Verification items for the finished model (mm, model axes). Face numbers are marked on the shaded views. Coordinates: 2 decimals unless noted, no trailing zeros. Order: outer loops, then holes, each group sorted by start corner. A loop starts at its lowest first (then second) coordinate and runs counter-clockwise, first axis right, second up. Notation, with made-up numbers: M 36,46.25 L 87,46.25 A17 ccw 87,62.25 Z; hole C -16.75,-27.5 d9. An arc over 180 degrees is marked long. Return JSON: item names as keys, results as strings. Group by question number.
Q1. Thickness scan on probe 1 along Z at (x, y) = (3, 23.5); probe 2 along Z at (x, y) = (-28, 0); probe 3 along Z at (x, y) = (22, -13.5). Record the ranges inside material, lowest first.
Q2. Section check A-A, the plane y = 0. Count the separate pieces of the cut face and the enclosed holes in it, then the cut area to 3 significant figures.
Q3. Go/stop test with flat-tipped pins: pin 1 Ø1.4 at (y, z) = (7.5, 54) entering from -X (3 decimals); pin 2 Ø2.5 at (y, z) = (20.5, -222) entering from -X; pin 3 Ø3.5 at (x, y) = (-1.5, 8.5) entering from +Z. Record where each tip stops, or that it passes through.
Q4. Mould release check, pull along Z, two halves, no side actions. Record for the marked faces 1 and 2: pulls with the +Z half, pulls with the -Z half, needs draft (parallel to the pull), parting line crosses it, or undercut.
Q5. Section check B-B, the plane y = 25.4. Enter the section's corners in (x, z).
Q6. Section check D-D, the plane z = -266.5. Enter the section's corners in (x, y), then the cut area to 3 significant figures.
Q7. Section check C-C, the plane z = -370.5. Enter the section's corners in (x, y) (3 decimals).
from build123d import *

# Parameters (mm, degrees)
BOSS_EXTRUDE1_DEPTH   = 5.08
LPATTERN1_COUNT       = 2
LPATTERN1_PITCH       = 104.14
SKETCH2_R             = 6.35
BOSS_EXTRUDE2_DEPTH   = 104.14
LPATTERN2_COUNT       = 3
LPATTERN2_PITCH       = 114.3
BODY_MOVE_COPY1_ANGLE = 120
BODY_MOVE_COPY2_ANGLE = 120
SKETCH3_R             = 12.7
BOSS_EXTRUDE3_DEPTH   = 5.08
BOSS_EXTRUDE4_START   = 114.3
SKETCH3_2_R           = 12.7
BOSS_EXTRUDE4_DEPTH   = 5.08
SKETCH4_R             = 6.985
BOSS_EXTRUDE5_DEPTH   = 76.2
SKETCH5_R             = 6.35
BOSS_EXTRUDE6_DEPTH   = 76.2
BOSS_EXTRUDE7_START   = 5.499261
SKETCH6_W             = 6.35
SKETCH6_H             = 25.4
BOSS_EXTRUDE7_DEPTH   = 4.660739


with BuildPart() as part:
    # Sketch1 → Boss-Extrude1 (new body)
    with BuildSketch(Plane.XY):
        with BuildLine():
            Line((15.24, 8.798818102), (15.24, 34.919226796))
            ThreePointArc((15.24, 34.919226796), (0, 38.1), (-15.24, 34.919226796))
            Line((-15.24, 34.919226796), (-15.24, 8.798818102))
            Line((-15.24, 8.798818102), (-37.860937485, -4.261386244))
            ThreePointArc((-37.860937485, -4.261386244), (0, -38.1), (37.860937485, -4.261386244))
            Line((37.860937485, -4.261386244), (15.24, 8.798818102))
        make_face()
    extrude(amount=-BOSS_EXTRUDE1_DEPTH)


with BuildPart() as lpattern1_1:
    # LPattern1: pattern copy
    add(part.part.moved(Location(Vector(0, 0, -1) * (1 * LPATTERN1_PITCH))))


with BuildPart() as part_1:
    add(part.part)

    add(lpattern1_1.part)  # Boss-Extrude2 merges LPattern1_1
    # Sketch2 → Boss-Extrude2 (add)
    with BuildSketch(Plane(origin=(0, 0, -5.08), x_dir=(-1, 0, 0), z_dir=(0, 0, -1))):
        with Locations((0, 25.4)):
            Circle(SKETCH2_R)
    extrude(amount=BOSS_EXTRUDE2_DEPTH)


with BuildPart() as lpattern2_1:
    # LPattern2: pattern copy
    add(part_1.part.moved(Location(Vector(0, 0, -1) * (1 * LPATTERN2_PITCH))))


with BuildPart() as lpattern2_2:
    # LPattern2: pattern copy
    add(part_1.part.moved(Location(Vector(0, 0, -1) * (2 * LPATTERN2_PITCH))))


with BuildPart() as lpattern2_1_1:
    # Body-Move/Copy1: moved
    add(lpattern2_1.part.rotate(Axis((0, 0, 0), (0, 0, 1)), BODY_MOVE_COPY1_ANGLE))


with BuildPart() as lpattern2_2_1:
    # Body-Move/Copy2: moved
    add(lpattern2_2.part.rotate(Axis((0, 0, 0), (0, 0, -1)), BODY_MOVE_COPY2_ANGLE))


with BuildPart() as part_2:
    add(part_1.part)

    add(lpattern2_1_1.part)  # Boss-Extrude3 merges LPattern2_1
    # Sketch3 → Boss-Extrude3 (add)
    with BuildSketch(Plane(origin=(0, 0, -109.22), x_dir=(-1, 0, 0), z_dir=(0, 0, -1))):
        Circle(SKETCH3_R)
    extrude(amount=BOSS_EXTRUDE3_DEPTH)

    add(lpattern2_2_1.part)  # Boss-Extrude4 merges LPattern2_2
    # Sketch3<2> → Boss-Extrude4 (add)
    with BuildSketch(Plane(origin=(0, 0, -109.22), x_dir=(-1, 0, 0), z_dir=(0, 0, -1)).offset(BOSS_EXTRUDE4_START)):
        Circle(SKETCH3_2_R)
    extrude(amount=BOSS_EXTRUDE4_DEPTH)

    # Sketch4 → Boss-Extrude5 (add)
    with BuildSketch(Plane(origin=(0, 0, -337.82), x_dir=(-1, 0, 0), z_dir=(0, 0, -1))):
        Circle(SKETCH4_R)
    extrude(amount=BOSS_EXTRUDE5_DEPTH)

    # Sketch5 → Boss-Extrude6 (add)
    with BuildSketch(Plane.XY):
        Circle(SKETCH5_R)
    extrude(amount=BOSS_EXTRUDE6_DEPTH)

    # Sketch6 → Boss-Extrude7 (add)
    with BuildSketch(Plane(origin=(0, 0, 0), x_dir=(1, 0, 0), z_dir=(0, 1, 0)).offset(BOSS_EXTRUDE7_START)):
        with Locations((0, -57.15)):
            Rectangle(SKETCH6_W, SKETCH6_H)
    extrude(amount=BOSS_EXTRUDE7_DEPTH)


solid = part_2.part
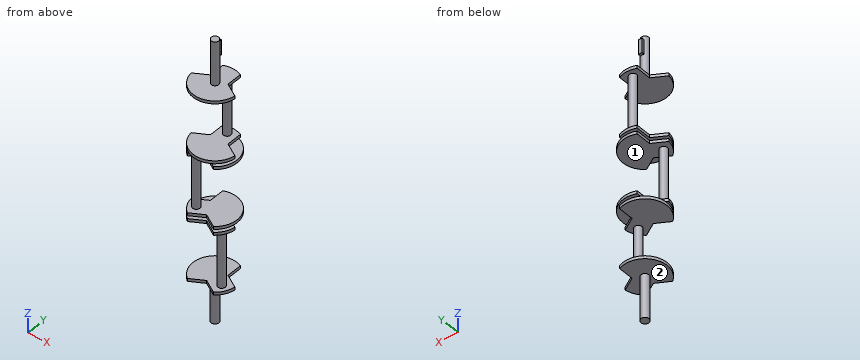
Numbers:
{
 "1": {"probe 1": "z = -337.82 to -332.74, -233.68 to -228.6, -223.52 to -218.44, -119.38 to -114.3, -109.22 to 0", "probe 2": "z = -337.82 to -332.74, -233.68 to -228.6, -223.52 to -218.44, -119.38 to -114.3, -109.22 to -104.14, -5.08 to 0", "probe 3": "z = -337.82 to -228.6, -223.52 to -218.44, -119.38 to -114.3, -109.22 to -104.14, -5.08 to 0"},
 "2": {"separate pieces": "4", "enclosed holes": "0", "area": "4,300 mm2"},
 "3": {"pin 1": "stops at x = -3.175", "pin 2": "stops at x = -15.24", "pin 3": "stops at z = 69.85"},
 "4": {"face 1": "undercut", "face 2": "pulls with the -Z half"},
 "5": {"outline": "M -28.4,-337.82 L 15.24,-337.82 L 15.24,-332.74 L -28.4,-332.74 Z; M -28.4,-233.68 L 15.24,-233.68 L 15.24,-228.6 L -28.4,-228.6 Z; M -15.24,-223.52 L 28.4,-223.52 L 28.4,-218.44 L -15.24,-218.44 Z; M -15.24,-119.38 L 28.4,-119.38 L 28.4,-114.3 L -15.24,-114.3 Z; M -15.24,-109.22 L 15.24,-109.22 L 15.24,-104.14 L 6.35,-104.14 L 6.35,-5.08 L 15.24,-5.08 L 15.24,0 L -15.24,0 L -15.24,-5.08 L -6.35,-5.08 L -6.35,-104.14 L -15.24,-104.14 Z"},
 "6": {"outline": "C 22,-12.7 d12.7", "area": "127 mm2"},
 "7": {"outline": "C 0,0 d13.97"}
}
